Design review of the part shown in the three views and the two pictorial views. Dimensions are in mm from the part's minimum x, y and z. Give positions to 0.01 mm unless a question says otherwise; leave off trailing zeros. Order: outer loops, then holes, each group sorted by start corner. A loop starts at its lowest first (then second) coordinate and runs counter-clockwise, first axis right, second up.
Item 1: Consider section B-B (z = 36). Give the boundary of the cut face in (x, y), plus the area to 3 significant figures.
Item 2: For probe 1 along X at (y, z) = (123.5, 15); probe 2 along Y at (x, z) = (1071, 5.5); probe 3 along Y at (x, z) = (1150.5, 44), list the stretches that pass through material, from the lowest coordinate up.
Item 3: Consider section A-A (x = 143). Give the boundary of the cut face in (y, z), plus the area to 3 significant figures.
Item 4: For P1, Ø15, axis at y = 132.5, z = 30, coming from the -X side; P2, Ø6, axis at y = 89, z = 19, coming from the -X side; P3, Ø3, axis at y = 189, z = 22, coming from the +X side, all flat-tipped, find the tip position at first contact; note any pin that passes through.
Item 5: Consider section D-D (y = 198.5). Give the boundary of the cut face in (x, z).
Item 6: Consider section C-C (y = 23). Give the boundary of the cut face in (x, z), plus the area to 3 significant figures.
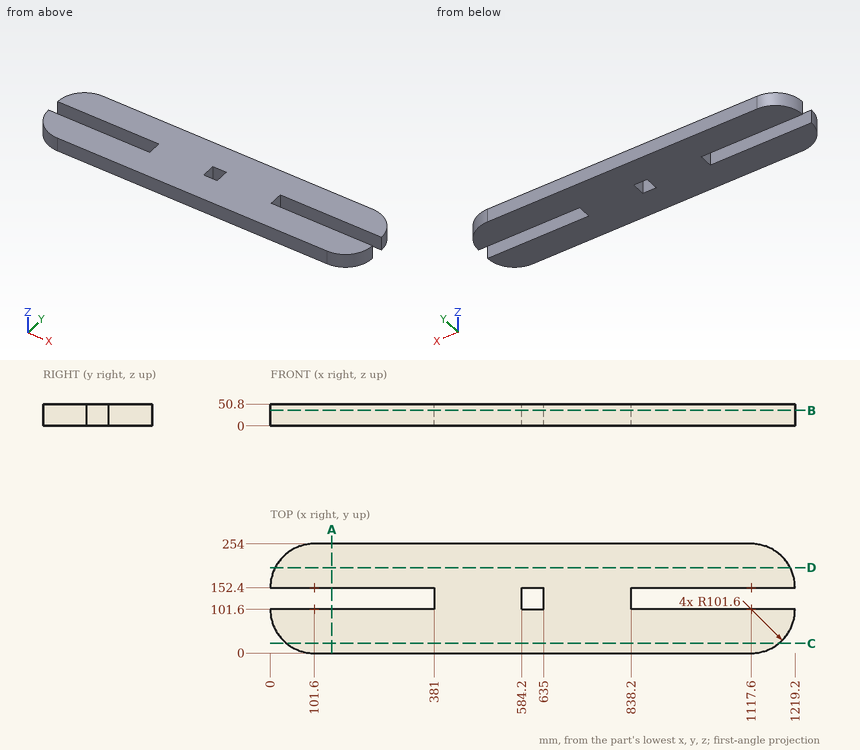
Resolved:
1. outline: (0, 101.6) arc R101.6 ccw to (101.6, 0) - (1117.6, 0) arc R101.6 ccw to (1219.2, 101.6) - (838.2, 101.6) - (838.2, 152.4) - (1219.2, 152.4) arc R101.6 ccw to (1117.6, 254) - (101.6, 254) arc R101.6 ccw to (0, 152.4) - (381, 152.4) - (381, 101.6) - close; hole (584.2, 101.6) - (635, 101.6) - (635, 152.4) - (584.2, 152.4) - close
1. area: 260,000 mm2
2. probe 1: x = 381 to 584.2, 635 to 838.2
2. probe 2: y = 0 to 101.6, 152.4 to 254
2. probe 3: y = 5.47 to 101.6, 152.4 to 248.53
3. outline: (0, 0) - (101.6, 0) - (101.6, 50.8) - (0, 50.8) - close; (152.4, 0) - (254, 0) - (254, 50.8) - (152.4, 50.8) - close
3. area: 10,300 mm2
4. P1: stops at x = 381
4. P2: stops at x = 0.45
4. P3: stops at x = 1212.94
5. outline: (11.06, 0) - (1208.14, 0) - (1208.14, 50.8) - (11.06, 50.8) - close
6. outline: (37.22, 0) - (1181.98, 0) - (1181.98, 50.8) - (37.22, 50.8) - close
6. area: 58,200 mm2
